```python
from build123d import *

# Parameters (mm, degrees)
CYLINDER043_R            = 1.65
CYLINDER043_DEPTH        = 10
CYLINDER044_R            = 1.65
CYLINDER044_DEPTH        = 10
BOX049_W                 = 32.25
BOX049_H                 = 42.5
BOX049_DEPTH             = 3
CHAMFER029006005013_SIZE = 0.4


with BuildPart() as cylinder043:
    # Cylinder043 → Cylinder043 (new body)
    with BuildSketch(Plane(origin=(24.25, 26, -13), x_dir=(1, 0, 0), z_dir=(0, 0, 1))):
        Circle(CYLINDER043_R)
    extrude(amount=CYLINDER043_DEPTH)


with BuildPart() as fusion006002011004053036004001_body:
    # Cylinder044 → Cylinder044 (new body)
    with BuildSketch(Plane(origin=(24.25, 60, -13), x_dir=(1, 0, 0), z_dir=(0, 0, 1))):
        Circle(CYLINDER044_R)
    extrude(amount=CYLINDER044_DEPTH)

    # Fusion006002011004053036004001028003011014: union Cylinder043
    add(cylinder043.part)


with BuildPart() as bottom_cover_r002:
    # Box049 → Box049 (new body)
    with BuildSketch(Plane(origin=(8, 21.75, -11), x_dir=(1, 0, 0), z_dir=(0, 0, 1))):
        with Locations((16.125, 21.25)):
            Rectangle(BOX049_W, BOX049_H)
    extrude(amount=BOX049_DEPTH)

    # Cut001024014003001002006005007: cut Fusion006002011004053036004001 body
    add(fusion006002011004053036004001_body.part, mode=Mode.SUBTRACT)

    # Chamfer029006005013
    chamfer029006005013_edges = [bottom_cover_r002.edges().sort_by_distance(p)[0] for p in [
        (8, 43, -11),
        (24.125, 21.75, -11),
        (24.125, 64.25, -11),
        (40.25, 43, -11),
        (22.6, 26, -11),
        (22.6, 60, -11),
    ]]
    chamfer(chamfer029006005013_edges, length=CHAMFER029006005013_SIZE)


solid = bottom_cover_r002.part
```
Verification items for the finished model (mm, model axes). Give positions to 0.01 mm unless a question says otherwise; leave off trailing zeros. Order: outer loops, then holes, each group sorted by start corner. A loop starts at its lowest first (then second) coordinate and runs counter-clockwise, first axis right, second up. Notation, with made-up numbers: (7, -21) -> (23, -21) arc R21 ccw to (23, -14) -> close; hole circle Ø11 at (50, 37.5). An arc over 180 degrees is marked (long way). One line per item, written item: value.
(1) Draft check along X on faces 1 (the face through (8, 43, -9)), 2 (the face through (24, 43, -11)), 3 (the face through (22.94, 59, -9.32)). Enter one of: pulls with the +X half, pulls with the -X half, needs draft (parallel to the pull), parting line crosses it, or undercut.
Final values:
face 1: pulls with the -X half
face 2: needs draft
face 3: undercut
(2) Sectioned sample at A-A on y = 26. Record the cut outline in (x, z), then the cut area to 3 significant figures.
Final values:
outline: (8, -10.6) -> (8.4, -11) -> (22.2, -11) -> (22.6, -10.6) -> (22.6, -8) -> (8, -8) -> close; (25.9, -10.6) -> (26.3, -11) -> (39.85, -11) -> (40.25, -10.6) -> (40.25, -8) -> (25.9, -8) -> close
area: 86.5 mm^2
(3) Gauge pin test, flat end, axial feed: pin 1 (3 mm diameter, centred on x = 24.25, y = 26, fed in from +Z). Record the tip position at first contact, or that the pin passes through.
Final values:
pin 1: through
(4) Scan lines: line 1 along Y through (x, z) = (24.25, -9.5); line 2 along X through (y, z) = (26, -9.1); line 3 along Y through (x, z) = (25, -8.6). Record each from-to range of solid material in increasing order. Write a range as [from, to].
Final values:
line 1: [21.75, 24.35], [27.65, 58.35], [61.65, 64.25]
line 2: [8, 22.6], [25.9, 40.25]
line 3: [21.75, 24.53], [27.47, 58.53], [61.47, 64.25]
(5) Sectioned sample at B-B on x = 24.25. Record the cut outline in (y, z).
Final values:
outline: (21.75, -10.6) -> (22.15, -11) -> (23.95, -11) -> (24.35, -10.6) -> (24.35, -8) -> (21.75, -8) -> close; (27.65, -10.6) -> (28.05, -11) -> (57.95, -11) -> (58.35, -10.6) -> (58.35, -8) -> (27.65, -8) -> close; (61.65, -10.6) -> (62.05, -11) -> (63.85, -11) -> (64.25, -10.6) -> (64.25, -8) -> (61.65, -8) -> close
